Check sheet for the drawn part. Datum: minimum x, y, z corner. Units: mm. Round coordinates to 2 decimals unless told otherwise and drop trailing zeros. Write each loop counter-clockwise with the first axis right and the second up, starting at its lowest first coordinate (ties: lowest second). Pieces come first, ordered by that corner, then holes. Notation, with made-up numbers: M -4.75,52.5 L 44.25,52.5 A34 ccw 44.25,85.5 Z; hole C 74,28.5 d11. An arc over 180 degrees is marked long. One line per item, written item: value.
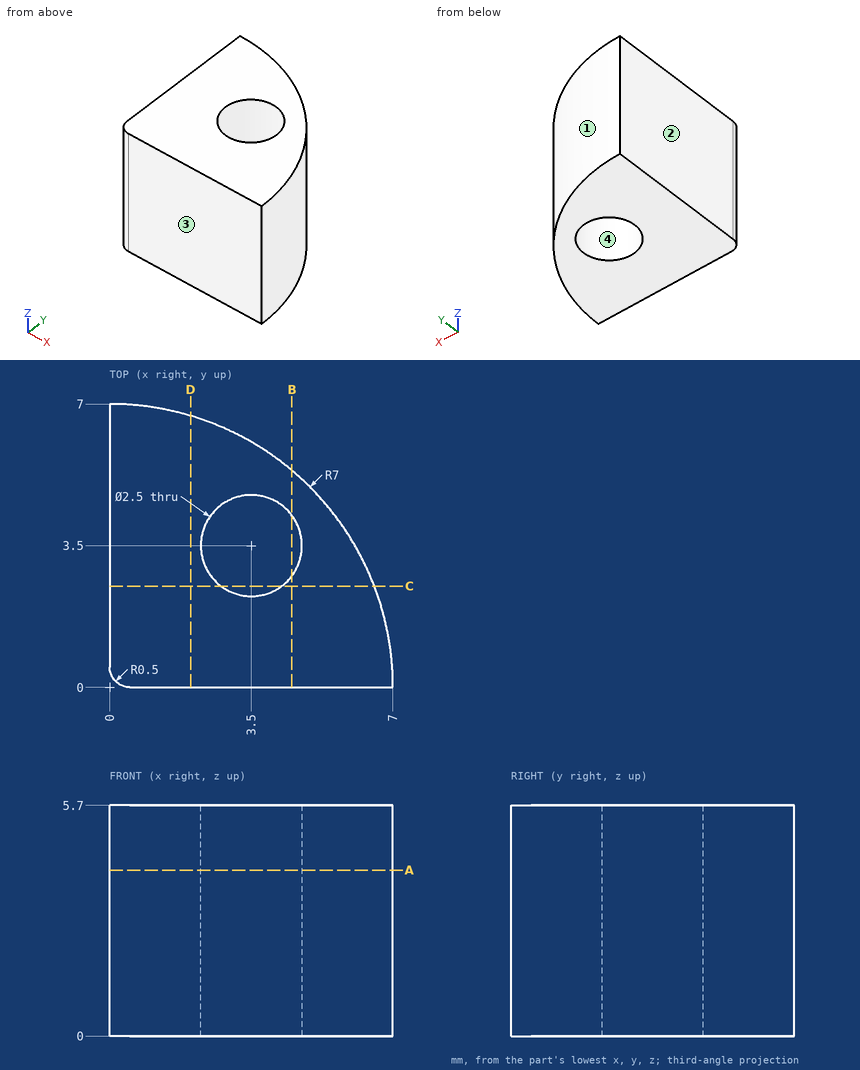
Q1. Sectioned sample at B-B on x = 4.5. Enter the section's corners in (y, z).
Completed:
outline: M 0,0 L 2.75,0 L 2.75,5.7 L 0,5.7 Z; M 4.25,0 L 5.36,0 L 5.36,5.7 L 4.25,5.7 Z
Q2. Sectioned sample at A-A on z = 4.1. Enter the section's corners in (x, y).
Completed:
outline: M 0,0.5 A0.5 ccw 0.5,0 L 7,0 A7 ccw 0,7 Z; hole C 3.5,3.5 d2.5
Q3. Scan lines: line 1 (Y direction, x = 4.25, z = 4.3); line 2 (Y direction, x = 3, z = 4.25) (1 decimal); line 3 (X direction, y = 4.5, z = 2.4). Record each from-to range of solid material in increasing order. Write a range as [from, to].
Completed:
line 1: [0, 2.5], [4.5, 5.56]
line 2: [0, 2.4], [4.6, 6.3]
line 3: [0, 2.75], [4.25, 5.36]
Q4. Sectioned sample at D-D on x = 2. Enter the section's corners in (y, z), and give its area (3 significant figures).
Completed:
outline: M 0,0 L 6.71,0 L 6.71,5.7 L 0,5.7 Z
area: 38.2 mm^2
Q5. Sectioned sample at C-C on y = 2.5. Enter the section's corners in (x, z), and give its area (3 significant figures).
Completed:
outline: M 0,0 L 2.75,0 L 2.75,5.7 L 0,5.7 Z; M 4.25,0 L 6.54,0 L 6.54,5.7 L 4.25,5.7 Z
area: 28.7 mm^2
Q6. Depth check by flat-ended pin: P1, Ø1.5, axis at y = 5.5, z = 0.5, coming from the +X side; P2, Ø3, axis at y = 3.5, z = 2, coming from the +X side; P3, Ø3, axis at x = 1.5, y = 6.5, coming from the -Z side. Enter the tip coordinate at first touch or a pass-through.
Completed:
P1: x = 5.14
P2: x = 6.71
P3: z = 0
Q7. Draft check along Y on the marked faces 1, 2, 3 and 4. Enter one of: pulls with the +Y half, pulls with the -Y half, needs draft (parallel to the pull), parting line crosses it, or undercut.
Completed:
face 1: pulls with the +Y half
face 2: needs draft
face 3: pulls with the -Y half
face 4: undercut
